from build123d import *

# Parameters (mm, degrees)
BOSS_EXTRUDE1_DEPTH = 30


with BuildPart() as part:
    # Sketch1 → Boss-Extrude1 (new body)
    with BuildSketch(Plane(origin=(0, 0, 0), x_dir=(0, 0, -1), z_dir=(1, 0, 0))):
        with BuildLine():
            Line((0, 0), (0, 29.130560593))
            ThreePointArc((0, 29.130560593), (5.792341896, 31.60023967), (10.990207869, 35.154494686))
            Line((10.990207869, 35.154494686), (30.714424781, 51.705077822))
            Line((30.714424781, 51.705077822), (32, 50.172988935))
            Line((32, 50.172988935), (2, 25))
            Line((2, 25), (2, 0))
            Line((2, 0), (0, 0))
        make_face()
    extrude(amount=BOSS_EXTRUDE1_DEPTH)


solid = part.part
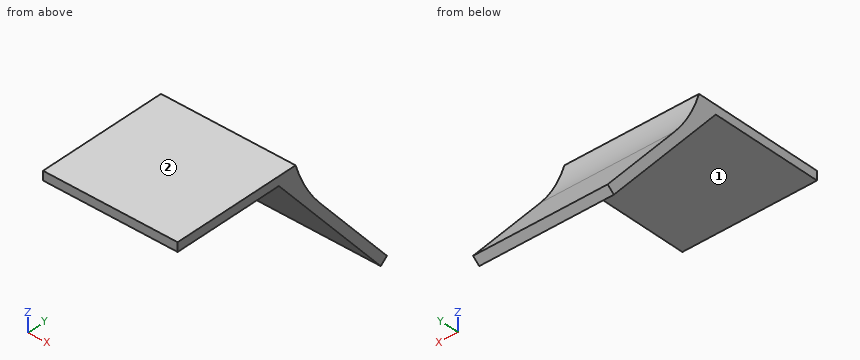
Could you check a few things on this model? Use its own coordinates, in mm. Face numbers are marked on the shaded views. A direction names the side the tool comes from. Give positions to 0.01 mm unless a question says otherwise; leave off trailing zeros. Order: outer loops, then holes, each group sorted by start corner. A loop starts at its lowest first (then second) coordinate and runs counter-clockwise, first axis right, second up.
1. Suppose I cut it at C-C (z = -19.5). List the corners of the cut face in (x, y) for me, plus the area to 3 significant figures.
2. I need wall thicknesses on L1, parallel to Z at x = 11.25, y = 4; L2, parallel to Y at x = 9.25, z = -18; L3, parallel to Y at x = 20.25, z = -12.5. Which ranges of each line are inside material? Lowest first, please.
3. Suppose I cut it at A-A (x = 11.75). List the corners of the cut face in (y, z) for me.
4. Suppose I cut it at B-B (y = 19). List the corners of the cut face in (x, z) for me.
5. Will these pins go through, and if not, where does the flat tip stop? P1, Ø2, axis at x = 20, z = -28.5, coming from the +Y side; P2, Ø10, axis at x = 12.5, z = -9.5, coming from the -Y side; P3, Ø2, axis at x = 9.5, y = 10.5, coming from the -Z side.
6. For the marked faces 1 and 2, which set-ups out of +Z, -Z, +X, -X, +Y, -Y let a thin tool reach every point of the face, with its end or its side?
Solved:
1. outline: (0, 39.68) - (30, 39.68) - (30, 42.3) - (0, 42.3) - close
1. area: 78.3 mm2
2. L1: z = -2 to 0
2. L2: y = 38.43 to 41.04
2. L3: y = 33.81 to 36.42
3. outline: (0, -2) - (25, -2) - (50.17, -32) - (51.71, -30.71) - (35.15, -10.99) arc R32.06 cw to (29.13, 0) - (0, 0) - close
4. outline: (0, -2) - (30, -2) - (30, 0) - (0, 0) - close
5. P1: stops at y = 50.69
5. P2: stops at y = 27.1
5. P3: stops at z = -2
6. face 1: -Z, +X, -X, -Y
6. face 2: +Z, +X, -X, +Y, -Y
